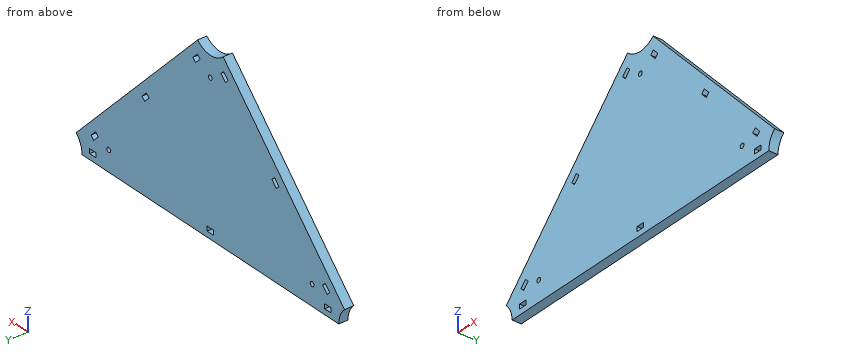
Autodesk Inventor part; units mm, degrees
ref_plane "YZ Plane" through (0, 0, 0) normal (1, 0, 0) x (0, 1, 0)
ref_plane "XZ Plane" through (0, 0, 0) normal (0, 1, 0) x (-1, 0, 0)
ref_plane "XY Plane" through (0, 0, 0) normal (0, 0, 1) x (1, 0, 0)
sketch "Sketch1" plane through (0, 0, 0) normal (0, 1, 0) x (-1, 0, 0)
  arc A0 (10, 0) -> (6.8806, 7.2566) centre (0, 0) ccw
  arc A1 (151.2194, 7.2566) -> (148.1, 0.0154) centre (158.1, 0) ccw
  circle A2 centre (79.05, 64.475) radius 1
  circle A3 centre (133.744, 8.9222) radius 1
  circle A4 centre (24.356, 8.9222) radius 1
  line L0 (6.8806, 7.2566) -> (72.1694, 76.1134)
  line L1 (85.9306, 76.1134) -> (151.2194, 7.2566)
  line L2 (148.1, 0.0154) -> (10, 0)
  arc A5 (72.1694, 76.1134) -> (85.9306, 76.1134) centre (79.05, 83.37) ccw
  line L3 (14.0684, 2.4018) -> (17.5684, 2.4018)
  line L4 (17.5684, 2.4018) -> (17.5684, 4.4018)
  line L5 (17.5684, 4.4018) -> (14.0684, 4.4018)
  line L6 (14.0684, 4.4018) -> (14.0684, 2.4018)
  line L7 (77.3084, 2.4018) -> (80.8084, 2.4018)
  line L8 (80.8084, 2.4018) -> (80.8084, 4.4018)
  line L9 (80.8084, 4.4018) -> (77.3084, 4.4018)
  line L10 (77.3084, 4.4018) -> (77.3084, 2.4018)
  line L11 (140.5484, 2.4018) -> (144.0484, 2.4018)
  line L12 (144.0484, 2.4018) -> (144.0484, 4.4018)
  line L13 (144.0484, 4.4018) -> (140.5484, 4.4018)
  line L14 (140.5484, 4.4018) -> (140.5484, 2.4018)
  line L15 (16.2824, 8.7713) -> (18.6906, 11.3111)
  line L16 (18.6906, 11.3111) -> (17.2392, 12.6872)
  line L17 (17.2392, 12.6872) -> (14.831, 10.1474)
  line L18 (14.831, 10.1474) -> (16.2824, 8.7713)
  line L19 (43.688, 37.6746) -> (46.0962, 40.2145)
  line L20 (46.0962, 40.2145) -> (44.6449, 41.5906)
  line L21 (44.6449, 41.5906) -> (42.2367, 39.0508)
  line L22 (42.2367, 39.0508) -> (43.688, 37.6746)
  line L23 (71.0937, 66.578) -> (73.5019, 69.1178)
  line L24 (73.5019, 69.1178) -> (72.0506, 70.4939)
  line L25 (72.0506, 70.4939) -> (69.6424, 67.9541)
  line L26 (69.6424, 67.9541) -> (71.0937, 66.578)
  line L27 (143.2789, 10.1369) -> (140.8707, 12.6767)
  line L28 (140.8707, 12.6767) -> (139.4194, 11.3006)
  line L29 (139.4194, 11.3006) -> (141.8276, 8.7608)
  line L30 (141.8276, 8.7608) -> (143.2789, 10.1369)
  line L31 (115.941, 38.9688) -> (113.5329, 41.5086)
  line L32 (113.5329, 41.5086) -> (112.0815, 40.1325)
  line L33 (112.0815, 40.1325) -> (114.4897, 37.5927)
  line L34 (114.4897, 37.5927) -> (115.941, 38.9688)
  line L35 (88.6032, 67.8006) -> (86.195, 70.3404)
  line L36 (86.195, 70.3404) -> (84.7437, 68.9643)
  line L37 (84.7437, 68.9643) -> (87.1519, 66.4245)
  line L38 (87.1519, 66.4245) -> (88.6032, 67.8006)
  point P0 (148.1, 0.0154)
  point P1 (151.2194, 7.2566)
  point P2 (85.9306, 76.1134)
extrude "Extrusion1" add sketch "Sketch1" along normal blind 4
properties part number "aab_face"
The model under review builds one solid part; all positions refer to its coordinate system, in mm. Coordinates: 2 decimals unless noted, no trailing zeros. Write each loop counter-clockwise with the first axis right and the second up, starting at its lowest first coordinate (ties: lowest second). Pieces come first, ordered by that corner, then holes.
1) We need section B-B on x = -83. State the section outline as (y, z) points, then the cut area to 3 significant figures.
2) Clearance check with flat-ended pins moving along their axes: pin 1 Ø1 at (x, y) = (-142.5, 3) entering from -Z; pin 2 Ø1 at (y, z) = (2, 3.5) entering from +X; pin 3 Ø1 at (y, z) = (3, 21) entering from +X; pin 4 Ø1.6 at (x, z) = (-24.36, 8.92) entering from +Y. State where each tip first meets the part, or that it passes through.
3) We need section C-C on z = 49. State the section outline as (x, y) points.
4) To check wall thickness, follow probe 1 along Z at (x, y) = (-79.05, 1.85) (3 decimals); probe 2 along X at (y, z) = (1.55, 39); probe 3 along X at (y, z) = (2.5, 10). State the ranges of each line that lie inside material, in increasing order.
5) We need section A-A on y = 2.4. Count the separate pieces of the cut face and the enclosed holes in it, then the cut area to 3 significant figures.
Answer list:
1. outline: (0, 0.01) - (4, 0.01) - (4, 74.18) - (0, 74.18) - close
1. area: 297 mm2
2. pin 1: stops at z = 0.01
2. pin 2: stops at x = -9.17
2. pin 3: stops at x = -19.44
2. pin 4: passes through
3. outline: (-111.64, 0) - (-46.46, 0) - (-46.46, 4) - (-111.64, 4) - close
4. probe 1: z = 0.008 to 2.402, 4.402 to 63.475, 65.475 to 73.37
4. probe 2: x = -121.12 to -115.91, -113.16 to -44.94, -42.29 to -36.98
4. probe 3: x = -148.62 to -143.13, -140.65 to -17.45, -14.99 to -9.48
5. separate pieces: 1
5. enclosed holes: 12
5. area: 6,360 mm2
